Verification items for the finished model (mm, model axes). Face numbers are marked on the shaded views. Coordinates: 2 decimals unless noted, no trailing zeros. Write each loop counter-clockwise with the first axis right and the second up, starting at its lowest first coordinate (ties: lowest second). Pieces come first, ordered by that corner, then holes. Notation, with made-up numbers: M 19.25,50 L 35.25,50 A9 cw 35.25,54 Z; hole C -14,-14 d3. An arc over 180 degrees is marked long. Answer in a Markdown table with one row per item.
from build123d import *
from OCP.BRepFilletAPI import BRepFilletAPI_MakeChamfer

# Parameters (mm, degrees)
ESQUISSE2_R                  = 26
BOSS_EXTRU_1_DEPTH           = 35
ESQUISSE3_R                  = 7.475
ENL_V_MAT_EXTRU_2_DEPTH      = 273.492201723
ENL_V_MAT_EXTRU_3_DEPTH      = 273.492201822
ENL_V_MAT_EXTRU_3_DEPTH_BACK = 273.492201822
ESQUISSE4_R                  = 10.125
BOSS_EXTRU_2_START           = -2.550056
ESQUISSE5_R                  = 11
ESQUISSE5_R_2                = 7.475
BOSS_EXTRU_2_DEPTH           = 2.550056
ESQUISSE6_R                  = 9.5
ESQUISSE6_R_2                = 7.475
BOSS_EXTRU_3_DEPTH           = 6
CHANFREIN2_SIZE              = 2
CHANFREIN2_SIZE2             = 1.453085056


with BuildPart() as part:
    # Esquisse1 → Révolution1 (revolve)
    with BuildSketch(Plane.XY):
        Polygon((0, 0), (25, 0), (25, 270), (12.5, 270), (12.5, 265), (20, 265), (20, 3), (0, 3), align=None)
    revolve(axis=Axis((0, 3, 0), (0, 1, 0)))

    # Esquisse2 → Boss.-Extru.1 (add)
    with BuildSketch(Plane(origin=(0, 0, 0), x_dir=(-1, 0, 0), z_dir=(0, -1, 0))):
        with Locations(Location((0, 0, 0), (0, 0, 180))):
            Circle(ESQUISSE2_R)
    extrude(amount=BOSS_EXTRU_1_DEPTH)

    # Esquisse3 → Enlèv. mat.-Extru.2 (cut, through all)
    with BuildSketch(Plane.XY):
        with Locations(Location((0, 11.5, 0), (0, 0, 180))):
            Circle(ESQUISSE3_R)
        with Locations(Location((0, 211.5, 0), (0, 0, 180))):
            Circle(ESQUISSE3_R)
    extrude(amount=ENL_V_MAT_EXTRU_2_DEPTH, mode=Mode.SUBTRACT)

    # Esquisse4 → Enlèv. mat.-Extru.3 (cut, two sides: drawn at the far end of the back side and taken through both)
    with BuildSketch(Plane(origin=(0, 0, 0), x_dir=(0, 0, -1), z_dir=(1, 0, 0)).offset(-ENL_V_MAT_EXTRU_3_DEPTH_BACK)):
        with Locations(Location((0, -17.5, 0), (0, 0, 270))):
            Circle(ESQUISSE4_R)
    extrude(amount=ENL_V_MAT_EXTRU_3_DEPTH + ENL_V_MAT_EXTRU_3_DEPTH_BACK, mode=Mode.SUBTRACT)

    # Esquisse5 → Boss.-Extru.2 (add)
    # profile 1 of 2: a face of its own
    with BuildSketch(Plane.XY.offset(25).offset(BOSS_EXTRU_2_START)):
        with Locations((0, 211.5)):
            Circle(ESQUISSE5_R)
        with Locations(Location((0, 211.5, 0), (0, 0, 180))):
            Circle(ESQUISSE5_R_2, mode=Mode.SUBTRACT)
    # profile 2 of 2: a face of its own
    with BuildSketch(Plane.XY.offset(25).offset(BOSS_EXTRU_2_START)):
        with Locations((0, 11.5)):
            Circle(ESQUISSE5_R)
        with Locations(Location((0, 11.5, 0), (0, 0, 180))):
            Circle(ESQUISSE5_R_2, mode=Mode.SUBTRACT)
    extrude(amount=BOSS_EXTRU_2_DEPTH)

    # Esquisse6 → Boss.-Extru.3 (add)
    # profile 1 of 2: a face of its own
    with BuildSketch(Plane.XY.offset(25)):
        with Locations((0, 211.5)):
            Circle(ESQUISSE6_R)
        with Locations(Location((0, 211.5, 0), (0, 0, 180))):
            Circle(ESQUISSE6_R_2, mode=Mode.SUBTRACT)
    # profile 2 of 2: a face of its own
    with BuildSketch(Plane.XY.offset(25)):
        with Locations((0, 11.5)):
            Circle(ESQUISSE6_R)
        with Locations(Location((0, 11.5, 0), (0, 0, 180))):
            Circle(ESQUISSE6_R_2, mode=Mode.SUBTRACT)
    extrude(amount=BOSS_EXTRU_3_DEPTH)

    # Chanfrein2: one chamfer whose edges measure the first distance from different faces: ONE call of the kernel's chamfer builder (chamfer() names one face for all edges)
    chanfrein2_edges_1 = [part.edges().sort_by_distance(p)[0] for p in [
        (6.717514421, 204.782485579, 25),
    ]]
    chanfrein2_side_1 = [part.faces().sort_by_distance(p)[0] for p in [
        (-9.5, 211.5, 28),
    ]]
    chanfrein2_edges_2 = [part.edges().sort_by_distance(p)[0] for p in [
        (6.717514421, 4.782485579, 25),
    ]]
    chanfrein2_side_2 = [part.faces().sort_by_distance(p)[0] for p in [
        (-9.5, 11.5, 28),
    ]]
    chanfrein2 = BRepFilletAPI_MakeChamfer(part.part.solid().wrapped)
    for e in chanfrein2_edges_1:
        chanfrein2.Add(CHANFREIN2_SIZE, CHANFREIN2_SIZE2, e.wrapped, chanfrein2_side_1[0].wrapped)  # the first distance lies on this face
    for e in chanfrein2_edges_2:
        chanfrein2.Add(CHANFREIN2_SIZE, CHANFREIN2_SIZE2, e.wrapped, chanfrein2_side_2[0].wrapped)  # the first distance lies on this face
    add(Compound.cast(chanfrein2.Shape()), mode=Mode.REPLACE)


solid = part.part
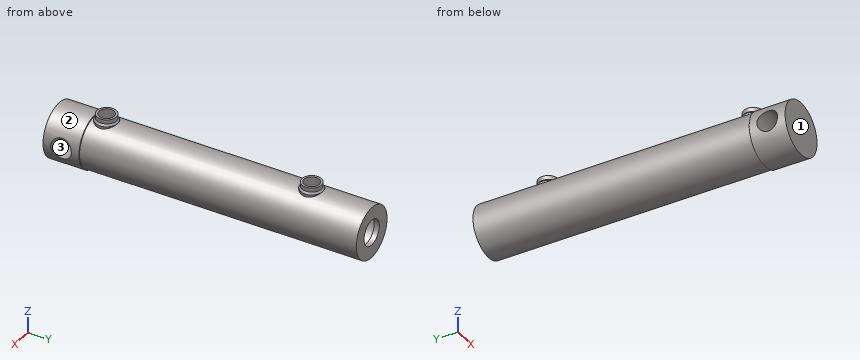
1) Sectioned sample at B-B (y = 11.5). Record the cut outline in (x, z) (3 decimals), then the cut area to 4 significant figures.
Response values:
| item | result |
|---|---|
| outline | M -11,22.45 A25 ccw long 11,22.45 L 11,25 L 10.953,25 L 9.5,27 L 9.5,31 L 7.475,31 L 7.475,18.551 A20 cw long -7.475,18.551 L -7.475,31 L -9.5,31 L -9.5,27 L -10.953,25 L -11,25 Z |
| area | 670.5 mm² |
2) Depth check by flat-ended pin: pin 1 (1.5 mm diameter, centred on y = 197, z = 3.5, fed in from -X); pin 2 (19.5 mm diameter, centred on x = 0, y = 211.5, fed in from +Z); pin 3 (2 mm diameter, centred on x = 18.5, y = 144, fed in from +Z); pin 4 (1.5 mm diameter, centred on y = 75, z = 16, fed in from +X). Enter the tip coordinate at first touch or a pass-through.
Response values:
| item | result |
|---|---|
| pin 1 | stops at x = -24.85 |
| pin 2 | stops at z = 31 |
| pin 3 | stops at z = 17.85 |
| pin 4 | stops at x = 19.81 |
3) Release check for a two-part mould opening along Z. For the marked faces 1, 2 and 3 record: +Z half, -Z half, draft (parallel to the pull), parting line (faces both ways), or undercut.
Response values:
| item | result |
|---|---|
| face 1 | draft |
| face 2 | parting line |
| face 3 | undercut |
4) Sectioned sample at C-C (y = 127.5). Record the cut outline in (x, z), then the cut area to 3 significant figures.
Response values:
| item | result |
|---|---|
| outline | C 0,0 d50; hole C 0,0 d40 |
| area | 707 mm² |
5) Sectioned sample at A-A (z = 0). Record the cut outline in (x, y) (3 decimals).
Response values:
| item | result |
|---|---|
| outline | M -26,-35 L 26,-35 L 26,-27.625 L -26,-27.625 Z; M -26,-7.375 L 26,-7.375 L 26,0 L 25,0 L 25,270 L 12.5,270 L 12.5,265 L 20,265 L 20,3 L -20,3 L -20,265 L -12.5,265 L -12.5,270 L -25,270 L -25,0 L -26,0 Z |
6) Thickness scan on L1, parallel to Y at x = 0, z = 22.5 (3 decimals); L2, parallel to Z at x = 0, y = 91. Record the ranges inside material, lowest first. Write a range as [from, to].
Response values:
| item | result |
|---|---|
| L1 | y = [-35, 4.025], [18.975, 204.025], [218.975, 270] |
| L2 | z = [-25, -20], [20, 25] |
